```python
from build123d import *

# Parameters (mm, degrees)
SKETCH2_R     = 4
CHAMFER1_SIZE = 0.5


with BuildPart() as part:
    # Sweep1: sweep along a path in Sketch1
    with BuildLine(Plane.XY) as sweep1_path:
        Line((-20, -58), (-20, 0))
        ThreePointArc((-20, 0), (0, 20), (20, 0))
        Line((20, 0), (20, -58))
    # Sketch2 → Sweep1 (sweep)
    with BuildSketch(Plane(origin=(0, -58, 0), x_dir=(1, 0, 0), z_dir=(0, 1, 0))):
        with Locations((-20, 0)):
            Circle(SKETCH2_R)
    sweep(path=sweep1_path.line)

    # Chamfer1
    chamfer1_edges = [part.edges().sort_by_distance(p)[0] for p in [
        (-24, -58, 0),
        (24, -58, 0),
    ]]
    chamfer(chamfer1_edges, length=CHAMFER1_SIZE)


solid = part.part
```
Work out the finished part from the listing and answer in its coordinate system (mm). A direction names the side the tool comes from. Round coordinates to 2 decimals unless told otherwise and drop trailing zeros. Write each loop counter-clockwise with the first axis right and the second up, starting at its lowest first coordinate (ties: lowest second). Pieces come first, ordered by that corner, then holes.
1) Flat-ended cylindrical pins translate along their axes: P1, Ø1.5, axis at y = -44, z = 1.5, coming from the +X side; P2, Ø3, axis at y = 11.5, z = 1, coming from the +X side; P3, Ø1.5, axis at x = -14, z = 1.5, coming from the -Y side. Find the tip coordinate at first contact, or state that the pin passes through.
2) A cutting plane is placed at B-B on z = 0. Determine the outline of the cut face in (x, y).
3) Consider probe 1 along X at (y, z) = (-2, -2.75); probe 2 along X at (y, z) = (-38, -0.25); probe 3 along Y at (x, z) = (-4, 1.5). Determine where each line is inside the solid, lowest interval first.
4) A cutting plane is placed at A-A on y = -11. Determine the outline of the cut face in (x, z).
5) Which of the six approach directions +Z, -Z, +X, -X, +Y, -Y give full straight-line access (tool end or side, diameter ignored) to faces 3 (the face through (23.2, -29.2, 2.4)), 4 (the face through (-20, -58, 0))?
6) Determine the mould class of faces 1 (the face through (20, -58, 0)), 2 (the face through (-23.2, -28.3, 2.4)) for opening direction X: pulls with the +X half, pulls with the -X half, needs draft (parallel to the pull), parting line crosses it, or undercut.
Entries:
1. P1: stops at x = 23.93
1. P2: stops at x = 21.74
1. P3: stops at y = 6.79
2. outline: (-24, -57.5) - (-23.5, -58) - (-16.5, -58) - (-16, -57.5) - (-16, 0) arc R16 cw to (16, 0) - (16, -57.5) - (16.5, -58) - (23.5, -58) - (24, -57.5) - (24, 0) arc R24 ccw to (-24, 0) - close
3. probe 1: x = -22.9 to -17.1, 17.1 to 22.9
3. probe 2: x = -23.99 to -16.01, 16.01 to 23.99
3. probe 3: y = 15.79 to 23.37
4. outline: circle Ø8 at (-20, 0); circle Ø8 at (20, 0)
5. face 3: -Y
5. face 4: +Z, -Z, +X, -X, -Y
6. face 1: needs draft
6. face 2: undercut
